Autodesk Fusion 360 part; units mm, degrees
sketch "Sketch1" plane through (0, 0, 0) normal (0, 1, 0) x (1, 0, 0)
  line L0 (-20.3838, 3.2056) -> (-17.6853, 3.2056)
  line L1 (-20.3584, -2.5911) -> (-17.8516, -2.5911)
  line L2 (-10.3249, 3.1994) -> (-0.7249, 3.1994)
  line L3 (-0.7249, 3.1994) -> (4.589, 0.1994)
  line L4 (4.589, 0.1994) -> (-0.7249, -2.8006)
  line L5 (-0.7249, -2.8006) -> (-10.3249, -2.8006)
  arc A0 (-20.1646, 3.2056) -> (-20.19, -2.5911) centre (-20.2742, 0.3077) ccw
  arc A1 (-10.3249, 3.1994) -> (-17.6853, 3.2056) centre (-14.0077, 0.1994) ccw
  arc A2 (-17.8516, -2.5911) -> (-10.3249, -2.8006) centre (-14.0077, 0.1994) ccw
  line L6 (-22.911, 1.5149) -> (3.7873, -2.43) construction
  dimension "d1" = 5.8
  dimension "d2" = 9.5
  dimension "d4" = 27.5
  dimension "d32" = 6
  dimension "d33" = 9.6
  dimension "d34" = 9
extrude "Extrude1" add sketch "Sketch1" along normal blind 8.2
sketch "Sketch2" plane through (0, 8.2, 0) normal (0, 1, 0) x (-1, 0, 0)
  arc A0 (20.3838, -3.2056) -> (20.3584, 2.5911) centre (20.2742, -0.3077) ccw
  line L0 (20.3584, 2.5911) -> (17.8516, 2.5911)
  arc A1 (17.8516, 2.5911) -> (10.3249, 2.8006) centre (14.0077, -0.1994) ccw
  line L1 (10.3249, 2.8006) -> (0.7249, 2.8006)
  line L2 (0.7249, 2.8006) -> (-4.589, -0.1994)
  line L3 (-4.589, -0.1994) -> (0.7249, -3.1994)
  line L4 (0.7249, -3.1994) -> (10.3249, -3.1994)
  arc A2 (10.3249, -3.1994) -> (17.6853, -3.2056) centre (14.0077, -0.1994) ccw
  line L5 (17.6853, -3.2056) -> (20.3838, -3.2056)
  circle A3 centre (14.0077, -0.1994) radius 3.3
  dimension "d9" = 6.6
extrude "Extrude2" cut sketch "Sketch2" against normal blind 5 contours A3
sketch "Sketch3" plane through (0, 3.2, 0) normal (0, 1, 0) x (-1, 0, 0)
  circle A0 centre (14.0077, -0.1994) radius 3.3
  line L0 (12.7077, -1.4994) -> (15.3077, -1.4994)
  line L1 (15.3077, -1.4994) -> (15.3077, 1.1006)
  line L2 (15.3077, 1.1006) -> (12.7077, 1.1006)
  line L3 (12.7077, 1.1006) -> (12.7077, -1.4994)
  line L4 (12.7077, -1.4994) -> (15.3077, 1.1006) construction
  line L5 (15.3077, -1.4994) -> (12.7077, 1.1006) construction
  point P0 (14.0077, -0.1994)
  dimension "d12" = 2.6
extrude "Extrude3" cut sketch "Sketch3" against normal blind 13 contours L0 L1 L2 L3
sketch "Sketch6" plane through (0, 8.2, 0) normal (0, 1, 0) x (-1, 0, 0)
  circle A0 centre (14.0077, -0.1994) radius 3.3
  arc A1 (20.3838, -3.2056) -> (20.3584, 2.5911) centre (20.2742, -0.3077) ccw
  line L0 (20.3584, 2.5911) -> (17.8516, 2.5911)
  arc A2 (17.8516, 2.5911) -> (10.3249, 2.8006) centre (14.0077, -0.1994) ccw
  line L1 (10.3249, 2.8006) -> (0.7249, 2.8006)
  line L2 (0.7249, 2.8006) -> (-4.589, -0.1994)
  line L3 (-4.589, -0.1994) -> (0.7249, -3.1994)
  line L4 (0.7249, -3.1994) -> (10.3249, -3.1994)
  arc A3 (10.3249, -3.1994) -> (17.6853, -3.2056) centre (14.0077, -0.1994) ccw
  line L5 (17.6853, -3.2056) -> (20.3838, -3.2056)
  line L6 (-0.0396, -2.1994) -> (9.9928, -2.1994) construction
  line L7 (9.9928, -2.1994) -> (9.9928, 1.8006) construction
  line L8 (9.9928, 1.8006) -> (-0.0396, 1.8006) construction
  line L9 (-0.0396, 1.8006) -> (-0.0396, -2.1994) construction
  line L10 (-0.0396, -2.1994) -> (9.9928, 1.8006) construction
  line L11 (9.9928, -2.1994) -> (-0.0396, 1.8006) construction
  line L12 (7.9828, 0.8006) -> (1.9704, 0.8006)
  line L13 (0.9604, -0.2094) -> (0.9604, -0.1894)
  line L14 (1.9704, -1.1994) -> (7.9828, -1.1994)
  line L15 (8.9928, -0.1894) -> (8.9928, -0.2094)
  arc A4 (0.9604, -0.1894) -> (1.9704, -1.1994) centre (1.9704, -0.1894) ccw
  arc A5 (1.9704, 0.8006) -> (0.9604, -0.2094) centre (1.9704, -0.2094) ccw
  arc A6 (8.9928, -0.2094) -> (7.9828, 0.8006) centre (7.9828, -0.2094) ccw
  arc A7 (7.9828, -1.1994) -> (8.9928, -0.1894) centre (7.9828, -0.1894) ccw
  line L16 (-4.589, -0.1994) -> (8.9928, -0.1994) construction
  line L17 (9.9928, -0.1994) -> (23.1722, -0.1994) construction
  point P0 (4.9766, -0.1994)
  dimension "d28" = 1.01
  dimension "d29" = 2
extrude "Extrude4" cut sketch "Sketch6" against normal blind 0.6 contours L12 L13 L14 L15 A4 A5 A6 A7
sketch "Sketch9" plane through (0, 0, 0) normal (0, -1, 0) x (1, 0, 0)
  line L0 (-12.7077, -1.4994) -> (-15.3077, -1.4994)
  line L1 (-15.3077, -1.4994) -> (-15.3077, 1.1006)
  line L2 (-15.3077, 1.1006) -> (-12.7077, 1.1006)
  line L3 (-12.7077, 1.1006) -> (-12.7077, -1.4994)
  arc A0 (-20.3584, 2.5911) -> (-20.3838, -3.2056) centre (-20.2742, -0.3077) ccw
  line L4 (-20.3838, -3.2056) -> (-17.6853, -3.2056)
  arc A1 (-17.6853, -3.2056) -> (-10.3249, -3.1994) centre (-14.0077, -0.1994) ccw
  line L5 (-10.3249, -3.1994) -> (-0.7249, -3.1994)
  line L6 (-0.7249, -3.1994) -> (4.589, -0.1994)
  line L7 (4.589, -0.1994) -> (-0.7249, 2.8006)
  line L8 (-0.7249, 2.8006) -> (-10.3249, 2.8006)
  arc A2 (-10.3249, 2.8006) -> (-17.8516, 2.5911) centre (-14.0077, -0.1994) ccw
  line L9 (-17.8516, 2.5911) -> (-20.3584, 2.5911)
  line L10 (-0.7249, -3.1994) -> (-10.3249, -3.1994)
  line L11 (-10.3249, 2.8006) -> (-0.7249, 2.8006)
  line L12 (-0.7249, 2.8006) -> (4.589, -0.1994)
  line L13 (4.589, -0.1994) -> (-0.7249, -3.1994)
  line L14 (-10.3249, -3.1994) -> (-10.3249, 2.8006) construction
  line L15 (-1.0403, -1.9994) -> (2.1481, -0.1994)
  line L16 (2.1481, -0.1994) -> (-1.0403, 1.6006)
  line L17 (-1.0403, 1.6006) -> (-9.1249, 1.6006)
  line L18 (-9.1249, -1.9994) -> (-9.1249, 1.6006)
  line L19 (-9.1249, -1.9994) -> (-1.0403, -1.9994)
  point P0 (-10.3249, -3.1994)
  point P1 (-0.7249, -3.1994)
  point P2 (4.589, -0.1994)
  point P3 (-0.7249, 2.8006)
  point P4 (-10.3249, 2.8006)
  dimension "d35" = -1.2
extrude "Extrude5" cut sketch "Sketch9" against normal blind 6 contours L15 L16 L17 L18 L19
fillet "Fillet1" radius 1.75 2 edges at (-9.1249, 3, 1.6006) (-9.1249, 3, -1.9994)
Work out the finished part from the listing and answer in its coordinate system (mm). A direction names the side the tool comes from. Coordinates: 2 decimals unless noted, no trailing zeros. Write each loop counter-clockwise with the first axis right and the second up, starting at its lowest first coordinate (ties: lowest second). Pieces come first, ordered by that corner, then holes.
Q1. A cutting plane is placed at C-C, the plane y = 6.25. Give the vertices of the cut face in (x, z).
Q2. A cutting plane is placed at B-B, the plane y = 2. Give the vertices of the cut face in (x, z).
Q3. Find the intervals of material crossed by line 1 (X direction, y = 5.5, z = -1); line 2 (Z direction, x = -3, y = 3); line 3 (X direction, y = 1.75, z = -1.25), in increasing order.
Q4. Determine the mould class of faces 6 (the face through (-19, 4, 2.591)), 7 (the face through (-12.708, 2, 0)), 8 (the face through (-14, 2, 1.101)), 9 (the face through (-14.06, 4.04, -4.95)) for opening direction Z: released by +Z, released by -Z, zero draft, split by the parting line, or undercut.
Q5. A cutting plane is placed at D-D, the plane x = -2.75. Give the vertices of the cut face in (y, z), then the cut area to 3 significant figures.
Q6. Each of these flat-tipped pins is pushed along its axis until it touches: pin 1 Ø0.7 at (x, y) = (-4.5, 8) entering from +Z; pin 2 Ø1.3 at (x, y) = (-19.5, 5) entering from +Z; pin 3 Ø4 at (x, y) = (-3.5, 2.5) entering from -Z. Where does it stop, or does it pass through?
Q7. Which of the six approach directions +Z, -Z, +X, -X, +Y, -Y give full straight-line access (tool end or side, diameter ignored) to faces 1 (the face through (-6, 4, -3.199)), 2 (the face through (-5, 4, 2.801)), 3 (the face through (-8.7, 7.9, 0.5)), 4 (the face through (-4, 3, -1.999)), 5 (the face through (-15.308, 2, 0))?
Q8. A cutting plane is placed at A-A, the plane x = -14. Give the vertices of the cut face in (y, z), then the cut area to 3 significant figures.
Findings below:
1. outline: (-20.38, -3.21) - (-17.69, -3.21) arc R4.75 ccw to (-10.32, -3.2) - (-0.72, -3.2) - (4.59, -0.2) - (-0.72, 2.8) - (-10.32, 2.8) arc R4.75 ccw to (-17.85, 2.59) - (-20.36, 2.59) arc R2.9 ccw to start; hole circle Ø6.6 at (-14.01, -0.2)
2. outline: (-20.38, -3.21) - (-17.69, -3.21) arc R4.75 ccw to (-10.32, -3.2) - (-0.72, -3.2) - (4.59, -0.2) - (-0.72, 2.8) - (-10.32, 2.8) arc R4.75 ccw to (-17.85, 2.59) - (-20.36, 2.59) arc R2.9 ccw to start; hole (-15.31, -1.5) - (-12.71, -1.5) - (-12.71, 1.1) - (-15.31, 1.1) - close; hole (-9.12, -0.25) arc R1.75 ccw to (-7.37, -2) - (-1.04, -2) - (2.15, -0.2) - (-1.04, 1.6) - (-7.37, 1.6) arc R1.75 ccw to (-9.12, -0.15) - close
3. line 1: x = -23.09 to -17.21, -10.81 to -8.96, 0.73 to 3.17
3. line 2: z = -3.2 to -2, 1.6 to 2.8
3. line 3: x = -23.02 to -15.31, -12.71 to -8.81, 0.29 to 2.73
4. face 6: released by +Z
4. face 7: undercut
4. face 8: undercut
4. face 9: released by -Z
5. outline: (0, -3.2) - (8.2, -3.2) - (8.2, -1.2) - (7.6, -1.2) - (7.6, 0.8) - (8.2, 0.8) - (8.2, 2.8) - (0, 2.8) - (0, 1.6) - (6, 1.6) - (6, -2) - (0, -2) - close
5. area: 26.4 mm2
6. pin 1: stops at z = 2.8
6. pin 2: stops at z = 2.59
6. pin 3: stops at z = -3.2
7. face 1: -Z, +X, +Y, -Y
7. face 2: +Z, +X, +Y, -Y
7. face 3: +Y
7. face 4: -Y
7. face 5: +Y, -Y
8. outline: (0, -4.95) - (8.2, -4.95) - (8.2, -3.5) - (3.2, -3.5) - (3.2, -1.5) - (0, -1.5) - close; (0, 1.1) - (3.2, 1.1) - (3.2, 3.1) - (8.2, 3.1) - (8.2, 4.55) - (0, 4.55) - close
8. area: 36.6 mm2
